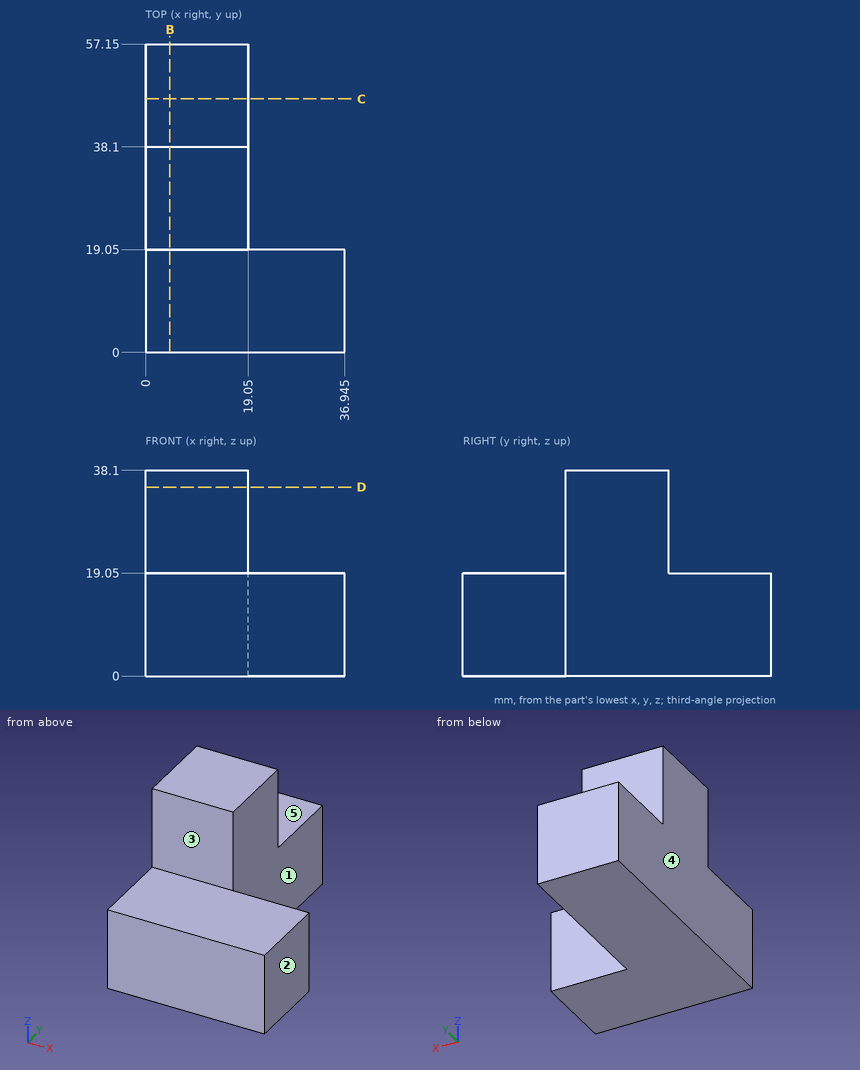
Check sheet for the drawn part. Datum: minimum x, y, z corner. Units: mm. A direction names the side the tool comes from. Round coordinates to 2 decimals unless told otherwise and drop trailing zeros. Loops run counter-clockwise (first coordinate to the right, second up) from the corner with the lowest first, then second, coordinate; pieces in that order, holes last. Notation, with made-up numbers: (2.5, 64) - (53.5, 64) arc R13 cw to (53.5, 78) - close; hole circle Ø8 at (8.5, 58.25). An arc over 180 degrees is marked (long way). Write item = value, one per line. Start each with the question number.
1. Section check C-C on y = 47. Enter the section's corners in (x, z), then the cut area to 3 significant figures.
2. Thickness scan on line 1 (Y direction, x = 28.5, z = 3); line 2 (Y direction, x = 17.5, z = 34). Record the ranges inside material, lowest first.
3. Section check D-D on z = 35. Enter the section's corners in (x, y).
4. Set-up check for the marked faces 1, 2, 3, 4 and 5: record each of +Z, -Z, +X, -X, +Y, -Y from which the full face is reachable in a straight line by a thin tool's end or side.
5. Depth check by flat-ended pin: pin 1 (1 mm diameter, centred on x = 5.5, z = 32.5, fed in from -Y); pin 2 (9.5 mm diameter, centred on x = 5, z = 30, fed in from +Y); pin 3 (5 mm diameter, centred on x = 32.5, z = 17, fed in from +Y); pin 4 (14.5 mm diameter, centred on x = 25.5, z = 13, fed in from +Y). Enter the tip coordinate at first touch or a pass-through.
6. Section check B-B on x = 4.5. Enter the section's corners in (y, z).
Working result:
q1.outline = (0, 0) - (19.05, 0) - (19.05, 19.05) - (0, 19.05) - close
q1.area = 363 mm^2
q2.line_1 = 0 to 19.05
q2.line_2 = 19.05 to 38.1
q3.outline = (0, 19.05) - (19.05, 19.05) - (19.05, 38.1) - (0, 38.1) - close
q4.face_1 = +Z, -Z, +X, +Y
q4.face_2 = +Z, -Z, +X, +Y, -Y
q4.face_3 = +Z, +X, -X, -Y
q4.face_4 = +Z, -Z, -X, +Y, -Y
q4.face_5 = +Z, +X, -X, +Y
q5.pin_1 = 19.05
q5.pin_2 = 38.1
q5.pin_3 = 19.05
q5.pin_4 = 57.15
q6.outline = (0, 0) - (57.15, 0) - (57.15, 19.05) - (38.1, 19.05) - (38.1, 38.1) - (19.05, 38.1) - (19.05, 19.05) - (0, 19.05) - close
